Autodesk Inventor part; units mm, degrees
ref_plane "YZ Plane" through (0, 0, 0) normal (1, 0, 0) x (0, 1, 0)
ref_plane "XZ Plane" through (0, 0, 0) normal (0, 1, 0) x (-1, 0, 0)
ref_plane "XY Plane" through (0, 0, 0) normal (0, 0, 1) x (1, 0, 0)
sketch "Esboço6" plane through (0, 0, 0) normal (0, 1, 0) x (-1, 0, 0)
  line L0 (0, -22) -> (-17, -22)
  line L1 (-22, -17) -> (-22, 17)
  line L2 (-17, 22) -> (17, 22)
  line L3 (22, 17) -> (22, -15.5)
  line L4 (15.5, -22) -> (0, -22)
  arc A0 (-22, -17) -> (-17, -22) centre (-17, -17) ccw
  arc A1 (-17, 22) -> (-22, 17) centre (-17, 17) ccw
  arc A2 (22, 17) -> (17, 22) centre (17, 17) ccw
  line L5 (15.5, -22) -> (17, -22)
  line L6 (22, -15.5) -> (22, -17)
  arc A3 (17, -22) -> (22, -17) centre (17, -17) ccw
  circle A4 centre (18.4142, -18.4142) radius 2
  circle A5 centre (18.4142, 18.4142) radius 2
  circle A6 centre (-18.4142, 18.4142) radius 2
  circle A7 centre (-18.4142, -18.4142) radius 2
  point P0 (0, 0)
  point P1 (-22, -22)
  point P2 (-22, 22)
  point P3 (22, 22)
  point P4 (22, -22)
  dimension "d23" = 22
  dimension "d24" = 22
  dimension "d25" = 44
  dimension "d26" = 44
  dimension "d28" = 5
  dimension "d29" = 5
  dimension "d31" = 4
  dimension "d35" = 4
  dimension "d36" = 4
  dimension "d37" = 4
extrude "Extrusão4" add sketch "Esboço6" along normal blind 1
sketch "Esboço7" plane through (0, 1, 0) normal (0, 1, 0) x (1, 0, 0)
  circle A0 centre (-18.4142, -18.4142) radius 2
  line L0 (-18.4142, -18.4142) -> (-16.4142, -18.4142)
  line L1 (-16.4142, -18.4142) -> (-16.4142, -19.4142)
  line L2 (-16.4142, -19.4142) -> (-15.4142, -19.4142)
  line L3 (-15.4142, -19.4142) -> (-0.4142, -19.4142)
  line L4 (-0.4142, -19.4142) -> (-0.4142, -12.4142)
  line L5 (-15.4142, -19.4142) -> (-15.4142, -12.4142)
  line L6 (-15.4142, -12.4142) -> (-0.4142, -12.4142)
  point P0 (0, 0)
  dimension "d40" = 1
  dimension "d41" = 1
  dimension "d42" = 15
  dimension "d43" = 7
extrude "Extrusão5" add sketch "Esboço7" along normal blind 9 contours L5 L6 L4 L3
chamfer "Chanfro1" distance 1.5 angle 45 2 edges at (-7.9142, 10, 19.4142) (-7.9142, 10, 12.4142)
sketch "Esboço8" plane through (0, 10, 0) normal (0, 1, 0) x (1, 0, 0)
  line L0 (-0.4142, -17.9142) -> (-0.4142, -13.9142)
  line L1 (-0.4142, -15.9142) -> (-15.4142, -15.9142)
  line L2 (-15.4142, -13.9142) -> (-15.4142, -17.9142)
  line L3 (-0.4142, -15.9142) -> (-5.4142, -15.9142)
  line L4 (-5.4142, -15.9142) -> (-10.4142, -15.9142)
  line L5 (-10.4142, -15.9142) -> (-15.4142, -15.9142)
  circle A0 centre (-2.9142, -15.9142) radius 1.5
  circle A1 centre (-7.9142, -15.9142) radius 1.5
  circle A2 centre (-12.9142, -15.9142) radius 1.5
  point P0 (0, 0)
  dimension "d49" = 5
  dimension "d50" = 5
  dimension "d51" = 3
  dimension "d52" = 3
  dimension "d53" = 3
extrude "Extrusão6" cut sketch "Esboço8" against normal blind 1
sketch "Esboço9" plane through (0, 1, 0) normal (0, 1, 0) x (1, 0, 0)
  circle A0 centre (18.4142, -18.4142) radius 2
  line L0 (18.4142, -18.4142) -> (16.4142, -18.4142)
  line L1 (16.4142, -18.4142) -> (16.4142, -19.4142)
  line L2 (16.4142, -19.4142) -> (15.4142, -19.4142)
  line L3 (15.4142, -19.4142) -> (0.4142, -19.4142)
  line L4 (0.4142, -19.4142) -> (0.4142, -14.4142)
  line L5 (0.4142, -14.4142) -> (15.4142, -14.4142)
  line L6 (15.4142, -14.4142) -> (15.4142, -19.4142)
  point P0 (0, 0)
  dimension "d56" = 1
  dimension "d57" = 1
  dimension "d58" = 15
  dimension "d59" = 5
extrude "Extrusão7" add sketch "Esboço9" along normal blind 7 contours L3 L4 L5 L6
sketch "Esboço11" plane through (0, 8, 0) normal (0, 1, 0) x (1, 0, 0)
  line L0 (0.4142, -19.4142) -> (0.4142, -14.4142)
  line L1 (0.4142, -19.4142) -> (0.4142, -14.4142)
  line L2 (0.4142, -14.4142) -> (0.4142, -16.9142)
  line L3 (0.4142, -16.9142) -> (15.4142, -16.9142)
  line L4 (15.4142, -19.4142) -> (15.4142, -14.4142)
  line L5 (0.4142, -19.4142) -> (0.4142, -16.9142)
  circle A0 centre (1.6642, -18.1642) radius 0.5
  circle A1 centre (4.1642, -18.1642) radius 0.5
  circle A2 centre (6.6642, -18.1642) radius 0.5
  circle A3 centre (9.1642, -18.1642) radius 0.5
  circle A4 centre (11.6642, -18.1642) radius 0.5
  circle A5 centre (14.1642, -18.1642) radius 0.5
  circle A6 centre (1.6642, -15.6642) radius 0.5
  circle A7 centre (4.1642, -15.6642) radius 0.5
  circle A8 centre (6.6642, -15.6642) radius 0.5
  circle A9 centre (9.1642, -15.6642) radius 0.5
  circle A10 centre (11.6642, -15.6642) radius 0.5
  circle A11 centre (14.1642, -15.6642) radius 0.5
  line L6 (15.4142, -14.4142) -> (0.4142, -14.4142)
  line L7 (0.4142, -14.4142) -> (15.4142, -14.4142)
  line L8 (15.4142, -14.4142) -> (15.4142, -16.9142)
  line L9 (15.4142, -19.4142) -> (15.4142, -16.9142)
  line L10 (0.4142, -14.4142) -> (0.4142, -19.4142)
  line L11 (0.4142, -19.4142) -> (15.4142, -19.4142)
  line L12 (0.4142, -19.4142) -> (15.4142, -19.4142)
  point P0 (0, 0)
  dimension "d68" = 1
  dimension "d69" = 1
  dimension "d70" = 1
  dimension "d71" = 1
  dimension "d72" = 1
  dimension "d73" = 1
extrude "Extrusão8" cut sketch "Esboço11" against normal blind 5
sketch "Esboço12" plane through (0, 1, 0) normal (0, 1, 0) x (1, 0, 0)
  circle A0 centre (-18.4142, -18.4142) radius 2
  line L0 (-18.4142, -9.4142) -> (-14.9142, -9.4142)
  line L1 (-14.9142, -9.4142) -> (-14.9142, 0.5858)
  line L2 (-14.9142, 0.5858) -> (-18.4142, 0.5858)
  line L3 (-22, 17) -> (-22, -17)
  line L4 (-18.4142, 0.5858) -> (-21.9142, 0.5858)
  line L5 (-21.9142, 0.5858) -> (-21.9142, -9.4142)
  line L6 (-21.9142, -9.4142) -> (-18.4142, -9.4142)
  point P0 (0, 0)
  dimension "d77" = 10
  dimension "d78" = 3.5
  dimension "d79" = 3.5
extrude "Extrusão9" add sketch "Esboço12" along normal blind 9 contours L6 L5 L4 L2 L1 L0
sketch "Esboço13" plane through (0, 10, 0) normal (0, 1, 0) x (1, 0, 0)
  line L0 (-14.9142, 0.5858) -> (-21.9142, 0.5858)
  line L1 (-18.4142, 0.5858) -> (-18.4142, -1.9142)
  line L2 (-18.4142, -1.9142) -> (-18.4142, -4.4142)
  line L3 (-18.4142, -4.4142) -> (-18.4142, -6.9142)
  circle A0 centre (-18.4142, -1.9142) radius 1.5
  circle A1 centre (-18.4142, -6.9142) radius 1.5
  point P0 (0, 0)
  point P1 (-16.9142, 0.5858)
  point P2 (-19.9142, 0.5858)
  dimension "d83" = 2.5
  dimension "d84" = 2.5
  dimension "d85" = 2.5
  dimension "d86" = 3
  dimension "d87" = 3
extrude "Extrusão10" cut sketch "Esboço13" against normal blind 1
chamfer "Chanfro2" distance 1.5 angle 45 2 edges at (-14.9142, 10, 4.4142) (-21.9142, 10, 4.4142)
sketch "Esboço14" plane through (0, 1, 0) normal (0, 1, 0) x (1, 0, 0)
  line L0 (-14.9142, 0.5858) -> (-14.9142, -9.4142)
  line L1 (-14.9142, -9.4142) -> (22, -9.4142)
  line L2 (22, -17) -> (22, 17)
  line L3 (-14.9142, 0.588) -> (22, 0.588)
  circle A0 centre (18.4142, -18.4142) radius 2
  line L4 (18.4142, -9.4142) -> (21.9142, -9.4142)
  line L5 (21.9142, -9.4142) -> (21.9142, 0.588)
  line L6 (18.4142, -9.4142) -> (14.9142, -9.4142)
  line L7 (14.9142, -9.4142) -> (14.9142, 0.588)
  line L8 (21.9142, 0.588) -> (14.9142, 0.588)
  point P0 (0, 0)
  dimension "d93" = 3.5
  dimension "d94" = 3.5
extrude "Extrusão11" add sketch "Esboço14" along normal blind 9 contours L7 L3 L5 L1
chamfer "Chanfro3" distance 1.5 angle 45 2 edges at (21.9142, 10, 4.4131) (14.9142, 10, 4.4131)
sketch "Esboço16" plane through (0, 10, 0) normal (0, 1, 0) x (1, 0, 0)
  circle A0 centre (-18.4142, -1.9142) radius 1.5
  line L0 (20.4142, 0.588) -> (20.4142, -9.4142)
  circle A1 centre (-18.4142, -6.9142) radius 1.5
  circle A2 centre (18.4142, -6.9142) radius 1.5
  circle A3 centre (18.4142, -1.9142) radius 1.5
  point P0 (0, 0)
  dimension "d101" = 3
  dimension "d102" = 3
extrude "Extrusão12" cut sketch "Esboço16" against normal blind 1 contours A2 | A3
sketch "Esboço17" plane through (0, 1, 0) normal (0, 1, 0) x (1, 0, 0)
  circle A0 centre (-18.4142, 18.4142) radius 2
  arc A1 (-17, 22) -> (-22, 17) centre (-17, 17) ccw
  circle A2 centre (18.4142, 18.4142) radius 2
  arc A3 (22, 17) -> (17, 22) centre (17, 17) ccw
  line L0 (-11.7958, 18.4142) -> (-11.7958, 22)
  line L1 (17, 22) -> (-17, 22)
  line L2 (11.7958, 18.4142) -> (11.7958, 22)
  line L3 (-11.7958, 22) -> (-11.7958, 7)
  line L4 (11.7958, 7) -> (11.7958, 22)
  line L5 (-11.7958, 22) -> (11.7958, 22)
  line L6 (-10.7958, 16) -> (10.7958, 16)
  line L7 (-11.2958, 16) -> (10.7958, 16)
  line L8 (10.7958, 16) -> (11.2958, 16)
  line L9 (-11.7958, 7) -> (-11.5458, 7)
  line L10 (-11.5458, 7) -> (-11.5458, 16)
  line L11 (-11.5458, 16) -> (-11.2958, 16)
  line L12 (11.7958, 7) -> (11.5458, 7)
  line L13 (11.5458, 7) -> (11.5458, 16)
  line L14 (11.5458, 16) -> (11.2958, 16)
  line L15 (-11.5458, 16.25) -> (-11.5458, 22)
  line L16 (-11.7958, 22) -> (-11.5458, 22)
  line L17 (11.5458, 16.25) -> (11.5458, 22)
  line L18 (7.2792, 16.25) -> (7.2792, 22)
  line L19 (7.2792, 22) -> (7.5292, 22)
  line L20 (7.5292, 22) -> (7.4542, 16.25)
  line L21 (3.8292, 16.25) -> (3.8292, 22)
  line L22 (3.8292, 22) -> (3.5792, 22)
  line L23 (3.5792, 22) -> (3.5792, 16.25)
  line L24 (0.0292, 16.25) -> (0.0292, 22)
  line L25 (0.0292, 22) -> (-0.2208, 22)
  line L26 (-0.2208, 22) -> (-0.2208, 16.25)
  line L27 (-4.1208, 16.25) -> (-4.1208, 22)
  line L28 (-4.1208, 22) -> (-3.8708, 22)
  line L29 (-3.8708, 22) -> (-3.8708, 16.25)
  line L30 (-7.5708, 16.25) -> (-7.5708, 22)
  line L31 (-7.5708, 22) -> (-7.8208, 22)
  line L32 (-7.8208, 22) -> (-7.8208, 16.25)
  line L33 (11.5458, 16.25) -> (7.4542, 16.25)
  line L34 (7.2792, 16.25) -> (3.8292, 16.25)
  line L35 (3.5792, 16.25) -> (0.0292, 16.25)
  line L36 (-0.2208, 16.25) -> (-3.8708, 16.25)
  line L37 (-4.1208, 16.25) -> (-7.5708, 16.25)
  line L38 (-7.8208, 16.25) -> (-11.5458, 16.25)
  point P0 (0, 0)
  dimension "d107" = 15
  dimension "d122" = 0.25
  dimension "d124" = 0.25
  dimension "d126" = 0.25
  dimension "d128" = 0.25
  dimension "d130" = 0.25
extrude "Extrusão13" add sketch "Esboço17" along normal blind 25 contours L0 L1 L15 L38 L32 L30 L37 L27 L29 L36 L26 L24 L35 L23 L21 L34 L18 L20 L33 L17 L2 L4 L12 L13 L14 L8 L6 L7 L11 L10 L9 L3
sketch "Esboço20" plane through (-11.5458, 1, -16) normal (0, 0, 1) x (1, 0, 0)
  line L0 (23.0917, 0) -> (0, 0)
  line L1 (11.575, 10) -> (0, 10.1493)
  line L2 (0, 0) -> (0, 25)
  line L3 (11.575, 10) -> (23.0917, 9.8514)
  line L4 (23.0917, 0) -> (23.0917, 25)
  line L5 (23.0917, 9.8514) -> (23.0917, 0)
  line L6 (23.0917, 0) -> (11.575, 0)
  line L7 (0, 10.1493) -> (0, 0)
  line L8 (11.575, 0) -> (15.125, 0)
  line L9 (0, 0) -> (11.575, 0)
  line L10 (11.575, 0) -> (0, 0)
  point P0 (11.5458, -1)
extrude "Extrusão14" add sketch "Esboço20" along normal blind 5
sketch "Esboço21" plane through (-11.5458, 26, -16) normal (0, 0, 1) x (1, 0, 0)
  line L0 (0, -14.8507) -> (0, -9.8507)
  line L1 (0, -14.8507) -> (0, 0)
  line L2 (0, -9.8507) -> (23.0917, -9.8507)
  line L3 (23.0917, -15.1486) -> (23.0917, 0)
  line L4 (23.0917, -9.8507) -> (23.0917, -15.1486)
  line L5 (23.0917, -15.1486) -> (0.4734, -14.8507)
  line L6 (0, -14.8507) -> (23.0917, -15.1486)
  line L7 (23.0917, -15.1486) -> (0, -14.8507)
  point P0 (11.5458, -26)
  dimension "d136" = 5
extrude "Extrusão15" add sketch "Esboço21" along normal blind 2.5
equation "\"Raio_vergadura\" = Espessura"
equation "\"Largura_alívio_de_vergadura\" = Espessura"
equation "\"Profundidade_alívio_de_vergadura\" = 0.5 * Espessura"
equation "\"Tamanho_alívio_de_dobra\" = 4 * Espessura"
equation "\"Remanescente_mínimo\" = 2 * Espessura"
equation "\"Raiodetransição\" = Raio_vergadura"
equation "\"Tamanho_de_raio_de_Jacobi\" = Raio_vergadura"
equation "\"TamanhoFolga\" = Espessura"
properties part number "Ponte_H" material "Alumínio 6061"
Check sheet for the modelled part. Datum: model origin and axes. Units: mm. A direction names the side the tool comes from. Give positions to 0.01 mm unless a question says otherwise; leave off trailing zeros. Write each loop counter-clockwise with the first axis right and the second up, starting at its lowest first coordinate (ties: lowest second). Pieces come first, ordered by that corner, then holes. Notation, with made-up numbers: (9.5, 3) -> (60.5, 3) arc R28 ccw to (60.5, 22) -> close; hole circle Ø10 at (58.25, 53). An arc over 180 degrees is marked (long way). Use one line per item in the form item = value. Start each with the question number.
1. Mould release check, pull along Z, two halves, no side actions. Record for faces 4 (the flat face through (-11.546, 16, -10)), 5 (the flat face through (-15.675, 9.26, 4.344)), 6 (the flat face through (0, 14, -13.5)): pulls with the +Z half, pulls with the -Z half, needs draft (parallel to the pull), parting line crosses it, or undercut.
2. Access from +Z, -Z, +X, -X, +Y, -Y to the whole of each face (thin tool, end or side, straight path). Record for faces 1 (the flat face through (-14.914, 5, 4)), 2 (the flat face through (-18, 9, 7)), 3 (the flat face through (-7.809, 9.26, 13.175)).
3. Thickness scan on line 1 along Z through (x, y) = (3, 2); line 2 along X through (y, z) = (6.75, 3.5); line 3 along Y through (x, z) = (-11, -17.5). Record the ranges inside material, lowest first. Write a range as from..to.
4. Section check C-C (x = -8.5). Record the cut outline in (y, z).
5. Section check B-B (z = -12.5). Record the cut outline in (x, y), and give its area (3 significant figures).
6. Go/stop test with flat-tipped pins: P1, Ø5.5, axis at x = 18, y = 5, coming from the +Z side; P2, Ø4, axis at x = -7.91, z = 15.91, coming from the +Y side; P3, Ø1.1, axis at x = -10, z = -19.5, coming from the +Y side. Record where each tip stops, or that it passes through.
7. Section check D-D (y = 6.5). Count the separate pieces of the cut face and the enclosed holes in it, and give its area (3 significant figures).
Conclusion:
q1.face_4 = undercut
q1.face_5 = needs draft
q1.face_6 = pulls with the +Z half
q2.face_1 = -Z, +Y
q2.face_2 = +Y
q2.face_3 = +X, -X, +Y
q3.line_1 = -16.25..-11, 14.41..19.41
q3.line_2 = -21.91..-14.91, 14.91..21.91
q3.line_3 = 0..1
q4.outline = (0, -22) -> (1, -22) -> (1, -16.25) -> (26, -16.25) -> (26, -16) -> (16.15, -16) -> (16.15, -13.5) -> (11.11, -13.5) -> (11.11, -11) -> (1, -11) -> (1, 12.41) -> (8.5, 12.41) -> (10, 13.91) -> (10, 14.53) -> (9, 14.53) -> (9, 17.3) -> (10, 17.3) -> (10, 17.91) -> (8.5, 19.41) -> (1, 19.41) -> (1, 22) -> (0, 22) -> close
q5.outline = (-22, 0) -> (22, 0) -> (22, 1) -> (11.8, 1) -> (11.8, 26) -> (11.55, 26) -> (11.55, 10.85) -> (0.03, 11) -> (-11.55, 11.15) -> (-11.55, 26) -> (-11.8, 26) -> (-11.8, 1) -> (-22, 1) -> close
q5.area = 287 mm²
q6.P1 = 9.41
q6.P2 = 10
q6.P3 = 1
q7.separate_pieces = 16
q7.enclosed_holes = 0
q7.area = 390 mm²
